Here's the drawing with two shaded views (mm, measured from the low corner). I have some questions. Coordinates: 2 decimals unless noted, no trailing zeros. Order: outer loops, then holes, each group sorted by start corner. A loop starts at its lowest first (then second) coordinate and runs counter-clockwise, first axis right, second up. Notation, with made-up numbers: M 53.5,-7 L 101.5,-7 A16 ccw 101.5,8 Z; hole C 57,-6 d10. An arc over 180 degrees is marked long. Put each result on its own line as item: value. Start each with the question number.
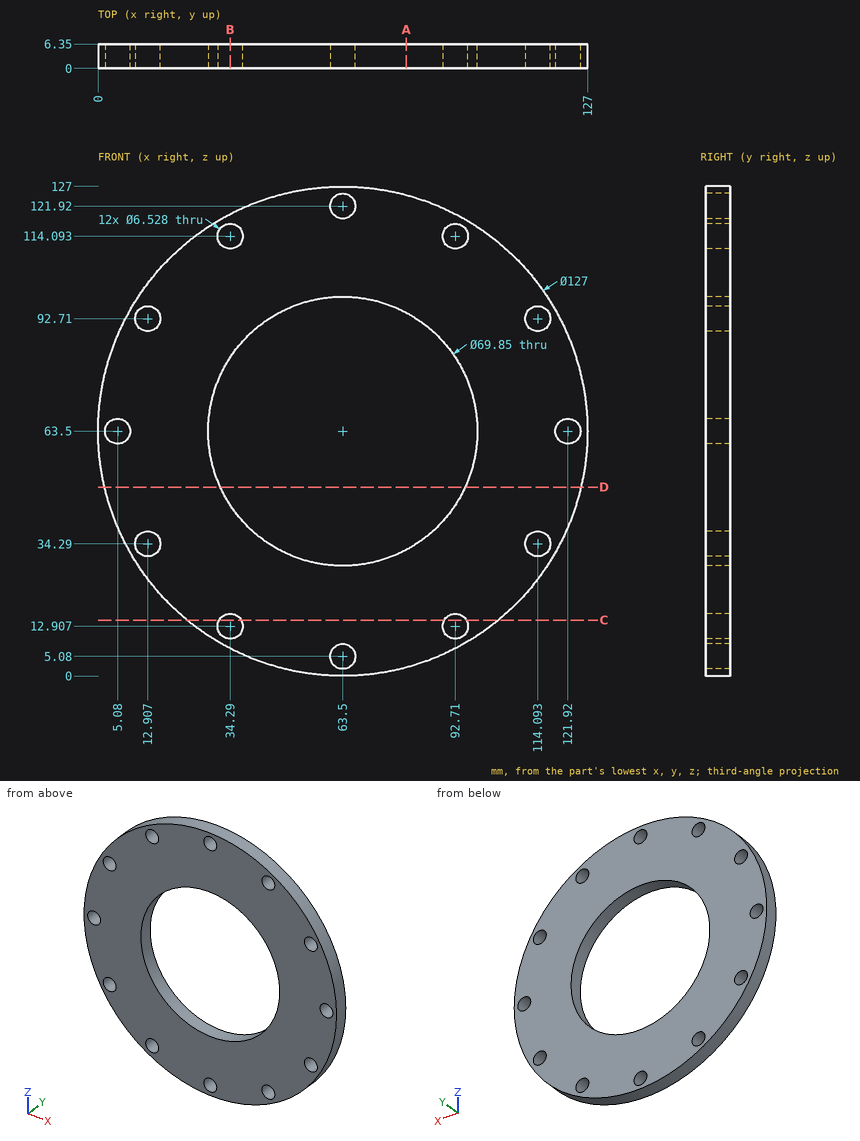
Item 1: For pin 1 Ø5 at (x, z) = (12.91, 92.71) entering from -Y; pin 2 Ø1 at (y, z) = (1.5, 102.5) entering from -X; pin 3 Ø1 at (x, y) = (111, 3.5) entering from -Z, each with a flat end and sliding along its axis, tell me the tip position at first contact or that it passes through.
Item 2: If we section it at D-D on z = 49: Write out the boundary of the cut face in (x, y).
Item 3: If we section it at B-B on x = 34.29: State how many separate pieces and enclosed holes the cut face has, then the cut area to 3 significant figures.
Item 4: If we section it at C-C on z = 14.5: Write out the boundary of the cut face in (x, y), then the cut area to 3 significant figures.
Item 5: I need wall thicknesses on probe 1 along X at (y, z) = (4.75, 62); probe 2 along X at (y, z) = (2.75, 35.5) (1 decimal); probe 3 along Z at (x, y) = (92.71, 3.5) (1 decimal). Which ranges of each line are inside material? Lowest first, please.
Item 6: If we section it at A-A on x = 80: Write out the boundary of the cut face in (y, z).
Geometry check:
1. pin 1: passes through
1. pin 2: stops at x = 13
1. pin 3: stops at z = 20.8
2. outline: M 1.68,0 L 31.73,0 L 31.73,6.35 L 1.68,6.35 Z; M 95.27,0 L 125.32,0 L 125.32,6.35 L 95.27,6.35 Z
3. separate pieces: 4
3. enclosed holes: 0
3. area: 390 mm²
4. outline: M 23.11,0 L 31.44,0 L 31.44,6.35 L 23.11,6.35 Z; M 37.14,0 L 89.86,0 L 89.86,6.35 L 37.14,6.35 Z; M 95.56,0 L 103.89,0 L 103.89,6.35 L 95.56,6.35 Z
4. area: 441 mm²
5. probe 1: x = 0.02 to 2.18, 7.98 to 28.61, 98.39 to 119.02, 124.82 to 126.98
5. probe 2: x = 6.5 to 9.9, 15.9 to 42.6, 84.4 to 111.1, 117.1 to 120.5
5. probe 3: z = 7.1 to 9.6, 16.2 to 44.4, 82.6 to 110.8, 117.4 to 119.9
6. outline: M 0,2.18 L 6.35,2.18 L 6.35,32.72 L 0,32.72 Z; M 0,94.28 L 6.35,94.28 L 6.35,124.82 L 0,124.82 Z
